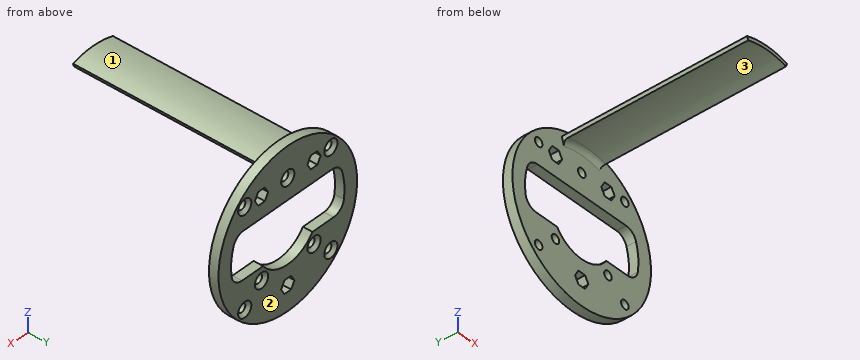
```python
from build123d import *

# Parameters (mm, degrees)
SKETCH1_R                                       = 33
SKETCH1_R_2                                     = 27
BOSS_EXTRUDE1_DEPTH                             = 4
SALIENTE_EXTRUIR1_START                         = -4
SKETCH2_R                                       = 1.5
SALIENTE_EXTRUIR1_DEPTH                         = 4
CORTAR_EXTRUIR1_REACH                           = 48.84
CROQUIS1_R                                      = 1.75
CSK_FOR_M3_FLAT_HEAD_MACHINE_SCREW1_D           = 3.6
CSK_FOR_M3_FLAT_HEAD_MACHINE_SCREW1_CSINK_D     = 6.3
CSK_FOR_M3_FLAT_HEAD_MACHINE_SCREW1_CSINK_ANGLE = 90
CSK_FOR_M3_FLAT_HEAD_MACHINE_SCREW2_D           = 3.6
CSK_FOR_M3_FLAT_HEAD_MACHINE_SCREW2_CSINK_D     = 6.3
CSK_FOR_M3_FLAT_HEAD_MACHINE_SCREW2_CSINK_ANGLE = 90
FILLET1_R                                       = 5
BOSS_EXTRUDE2_DEPTH                             = 78
FILLET2_R                                       = 2


with BuildPart() as part:
    # Sketch1 → Boss-Extrude1 (new body)
    with BuildSketch(Plane(origin=(0, 0, 0), x_dir=(1, 0, 0), z_dir=(0, 1, 0))):
        with Locations(Location((0, 0, 0), (0, 0, 270))):
            Circle(SKETCH1_R)
        with Locations(Location((0, 0, 0), (0, 0, 270))):
            Circle(SKETCH1_R_2, mode=Mode.SUBTRACT)
    extrude(amount=BOSS_EXTRUDE1_DEPTH)

    # Sketch2 → Saliente-Extruir1 (add)
    # profile 1 of 2: a face of its own
    with BuildSketch(Plane(origin=(0, 4, 0), x_dir=(1, 0, 0), z_dir=(0, 1, 0)).offset(SALIENTE_EXTRUIR1_START)):
        with BuildLine():
            Line((-24.5, -11.346805718), (24.5, -11.346805718))
            ThreePointArc((24.5, -11.346805718), (0, -27), (-24.5, -11.346805718))
        make_face()
        with Locations(Location((0, -20.2, 0), (0, 0, 270))):
            Circle(SKETCH2_R, mode=Mode.SUBTRACT)
    # profile 2 of 2: a face of its own
    with BuildSketch(Plane(origin=(0, 4, 0), x_dir=(1, 0, 0), z_dir=(0, 1, 0)).offset(SALIENTE_EXTRUIR1_START)):
        with BuildLine():
            Line((-25.7325, 8.175478197), (-11.7325, 8.175478197))
            ThreePointArc((-11.7325, 8.175478197), (0, 14.3), (11.7325, 8.175478197))
            Line((11.7325, 8.175478197), (25.7325, 8.175478197))
            ThreePointArc((25.7325, 8.175478197), (0, 27), (-25.7325, 8.175478197))
        make_face()
        with Locations(Location((-12.5, 13.5, 0), (0, 0, 270))):
            Circle(SKETCH2_R, mode=Mode.SUBTRACT)
        with Locations(Location((12.5, 13.5, 0), (0, 0, 270))):
            Circle(SKETCH2_R, mode=Mode.SUBTRACT)
    extrude(amount=SALIENTE_EXTRUIR1_DEPTH)

    # Croquis1 → Cortar-Extruir1 (cut, up to next)
    with BuildSketch(Plane(origin=(0, 4, 0), x_dir=(1, 0, 0), z_dir=(0, 1, 0)), mode=Mode.PRIVATE) as cortar_extruir1_sk1:
        with Locations(Location((-20.506096654, 20.506096654, 0), (0, 0, 270))):
            Circle(CROQUIS1_R)
    cortar_extruir1_tool1 = extrude(cortar_extruir1_sk1.sketch, amount=-CORTAR_EXTRUIR1_REACH, mode=Mode.PRIVATE) & part.part
    # Croquis1 → Cortar-Extruir1 (cut, up to next)
    with BuildSketch(Plane(origin=(0, 4, 0), x_dir=(1, 0, 0), z_dir=(0, 1, 0)), mode=Mode.PRIVATE) as cortar_extruir1_sk2:
        with Locations(Location((20.506096654, 20.506096654, 0), (0, 0, 270))):
            Circle(CROQUIS1_R)
    cortar_extruir1_tool2 = extrude(cortar_extruir1_sk2.sketch, amount=-CORTAR_EXTRUIR1_REACH, mode=Mode.PRIVATE) & part.part
    # Croquis1 → Cortar-Extruir1 (cut, up to next)
    with BuildSketch(Plane(origin=(0, 4, 0), x_dir=(1, 0, 0), z_dir=(0, 1, 0)), mode=Mode.PRIVATE) as cortar_extruir1_sk3:
        with Locations(Location((-20.506096654, -20.506096654, 0), (0, 0, 270))):
            Circle(CROQUIS1_R)
    cortar_extruir1_tool3 = extrude(cortar_extruir1_sk3.sketch, amount=-CORTAR_EXTRUIR1_REACH, mode=Mode.PRIVATE) & part.part
    # Croquis1 → Cortar-Extruir1 (cut, up to next)
    with BuildSketch(Plane(origin=(0, 4, 0), x_dir=(1, 0, 0), z_dir=(0, 1, 0)), mode=Mode.PRIVATE) as cortar_extruir1_sk4:
        with Locations(Location((20.506096654, -20.506096654, 0), (0, 0, 270))):
            Circle(CROQUIS1_R)
    cortar_extruir1_tool4 = extrude(cortar_extruir1_sk4.sketch, amount=-CORTAR_EXTRUIR1_REACH, mode=Mode.PRIVATE) & part.part
    # Croquis1 → Cortar-Extruir1 (cut, up to next)
    with BuildSketch(Plane(origin=(0, 4, 0), x_dir=(1, 0, 0), z_dir=(0, 1, 0)), mode=Mode.PRIVATE) as cortar_extruir1_sk5:
        Polygon((-9.324573519, -20), (-10.91228676, -17.25), (-14.08771324, -17.25), (-15.675426481, -20), (-14.08771324, -22.75), (-10.91228676, -22.75), align=None)
    cortar_extruir1_tool5 = extrude(cortar_extruir1_sk5.sketch, amount=-CORTAR_EXTRUIR1_REACH, mode=Mode.PRIVATE) & part.part
    # Croquis1 → Cortar-Extruir1 (cut, up to next)
    with BuildSketch(Plane(origin=(0, 4, 0), x_dir=(1, 0, 0), z_dir=(0, 1, 0)), mode=Mode.PRIVATE) as cortar_extruir1_sk6:
        Polygon((15.675426481, -20), (14.08771324, -17.25), (10.91228676, -17.25), (9.324573519, -20), (10.91228676, -22.75), (14.08771324, -22.75), align=None)
    cortar_extruir1_tool6 = extrude(cortar_extruir1_sk6.sketch, amount=-CORTAR_EXTRUIR1_REACH, mode=Mode.PRIVATE) & part.part
    # Croquis1 → Cortar-Extruir1 (cut, up to next)
    with BuildSketch(Plane(origin=(0, 4, 0), x_dir=(1, 0, 0), z_dir=(0, 1, 0)), mode=Mode.PRIVATE) as cortar_extruir1_sk7:
        Polygon((3.175426481, 22.5), (1.58771324, 25.25), (-1.58771324, 25.25), (-3.175426481, 22.5), (-1.58771324, 19.75), (1.58771324, 19.75), align=None)
    cortar_extruir1_tool7 = extrude(cortar_extruir1_sk7.sketch, amount=-CORTAR_EXTRUIR1_REACH, mode=Mode.PRIVATE) & part.part
    add(cortar_extruir1_tool1.solids().sort_by_distance((-20.506097, 4, -20.506097))[0], mode=Mode.SUBTRACT)
    add(cortar_extruir1_tool2.solids().sort_by_distance((20.506097, 4, -20.506097))[0], mode=Mode.SUBTRACT)
    add(cortar_extruir1_tool3.solids().sort_by_distance((-20.506097, 4, 20.506097))[0], mode=Mode.SUBTRACT)
    add(cortar_extruir1_tool4.solids().sort_by_distance((20.506097, 4, 20.506097))[0], mode=Mode.SUBTRACT)
    add(cortar_extruir1_tool5.solids().sort_by_distance((-12.5, 4, 20))[0], mode=Mode.SUBTRACT)
    add(cortar_extruir1_tool6.solids().sort_by_distance((12.5, 4, 20))[0], mode=Mode.SUBTRACT)
    add(cortar_extruir1_tool7.solids().sort_by_distance((0, 4, -22.5))[0], mode=Mode.SUBTRACT)

    # CSK for M3 Flat Head Machine Screw1 (through all)
    with Locations(Plane(origin=(0, 4, 0), x_dir=(1, 0, 0), z_dir=(0, 1, 0))):
        with Locations((-20.506096654, 20.506096654), (20.506096654, 20.506096654), (20.506096654, -20.506096654), (-20.506096654, -20.506096654)):
            CounterSinkHole(CSK_FOR_M3_FLAT_HEAD_MACHINE_SCREW1_D / 2, CSK_FOR_M3_FLAT_HEAD_MACHINE_SCREW1_CSINK_D / 2, counter_sink_angle=CSK_FOR_M3_FLAT_HEAD_MACHINE_SCREW1_CSINK_ANGLE)

    # CSK for M3 Flat Head Machine Screw2 (through all)
    with Locations(Plane(origin=(0, 4, 0), x_dir=(1, 0, 0), z_dir=(0, 1, 0))):
        with Locations((-12.5, 13.5), (12.5, 13.5), (0, -20.2)):
            CounterSinkHole(CSK_FOR_M3_FLAT_HEAD_MACHINE_SCREW2_D / 2, CSK_FOR_M3_FLAT_HEAD_MACHINE_SCREW2_CSINK_D / 2, counter_sink_angle=CSK_FOR_M3_FLAT_HEAD_MACHINE_SCREW2_CSINK_ANGLE)

    # Fillet1
    fillet1_edges = [part.edges().sort_by_distance(p)[0] for p in [
        (-25.7325, 2, -8.175478197),
        (25.7325, 2, -8.175478197),
        (24.5, 2, 11.346805718),
        (-24.5, 2, 11.346805718),
    ]]
    fillet(fillet1_edges, radius=FILLET1_R)

    # Sketch8 → Boss-Extrude2 (add)
    with BuildSketch(Plane(origin=(0, 0, 0), x_dir=(-1, 0, 0), z_dir=(0, -1, 0))):
        with BuildLine():
            Line((-9.486821727, -29.19743505), (-9.023296236, -27.770850276))
            ThreePointArc((-9.023296236, -27.770850276), (0, -29.2), (9.023296236, -27.770850276))
            Line((9.023296236, -27.770850276), (9.486821727, -29.19743505))
            ThreePointArc((9.486821727, -29.19743505), (0, -30.7), (-9.486821727, -29.19743505))
        make_face()
    extrude(amount=BOSS_EXTRUDE2_DEPTH)

    # Fillet2
    fillet2_edges = [part.edges().sort_by_distance(p)[0] for p in [
        (0, 0, 29.2),
    ]]
    fillet(fillet2_edges, radius=FILLET2_R)


solid = part.part
```
Here's how the part is built. I have some questions about the finished solid (model axes, mm). Face numbers are marked on the shaded views. A direction names the side the tool comes from. Coordinates: 2 decimals unless noted, no trailing zeros. Order: outer loops, then holes, each group sorted by start corner. A loop starts at its lowest first (then second) coordinate and runs counter-clockwise, first axis right, second up. Notation, with made-up numbers: (53, 39.25) - (105, 39.25) arc R11 ccw to (105, 56.25) - close; hole circle Ø2 at (-16, -10.5). An arc over 180 degrees is marked (long way). One line per question, with ' | ' between items. Start each with the question number.
1. Please list where these lines run through material, in increasing order: line 1 along X through (y, z) = (2, -13); line 2 along Y through (x, z) = (5.5, 24); line 3 along Z through (x, y) = (-4, -47). Write a range as [from, to].
2. Which directions (+Z, -Z, +X, -X, +Y, -Y) give clear straight access to the entire face, cutting with the end or side of a thin tool? Please do the marked faces 1, 2 and 3.
3. If we section it at C-C (y = -64.5): Write out the boundary of the cut face in (x, z).
4. If we section it at A-A (z = 0): Write out the boundary of the cut face in (x, y).
5. I'm going to push flat-ended pins straight in: pin 1 Ø3 at (x, z) = (-20.51, 20.51) entering from -Y; pin 2 Ø6 at (x, z) = (12.5, -13.5) entering from -Y; pin 3 Ø1 at (x, y) = (-13.5, 2.5) entering from -Z; pin 4 Ø2.5 at (x, y) = (12.5, 2) entering from -Z. Where does each tip first touch, or does it pass through?
6. If we section it at B-B (x = 0): Give the number of separate pieces and of enclosed holes in the cut face, and give its area (3 significant figures).
Model answer:
1) line 1: x = [-30.33, -14.23], [-10.77, -5.96], [5.96, 10.77], [14.23, 30.33] | line 2: y = [0, 4] | line 3: z = [28.92, 30.44]
2) face 1: +Z, -Y | face 2: +Z, -Z, +X, -X, +Y | face 3: -Z, -Y
3) outline: (-9.49, 29.2) - (-9.02, 27.77) arc R29.2 cw to (9.02, 27.77) - (9.49, 29.2) arc R30.7 ccw to start
4) outline: (-33, 0) - (-27, 0) - (-27, 4) - (-33, 4) - close; (27, 0) - (33, 0) - (33, 4) - (27, 4) - close
5) pin 1: passes through | pin 2: stops at y = 0 | pin 3: stops at z = -30.33 | pin 4: stops at z = -31.02
6) separate pieces: 4 | enclosed holes: 0 | area: 241 mm²
